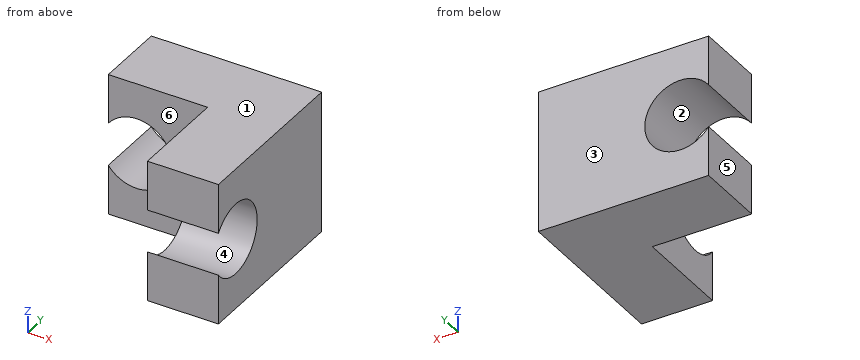
```python
from build123d import *

# Parameters (mm, degrees)
F1_DEPTH       = 12.7
F4_D           = 6.35
F4_DEPTH       = 25.4
F4_TIP         = 1.9077324654
F4_ON_F3_D     = 6.35
F4_ON_F3_DEPTH = 25.4
F4_ON_F3_TIP   = 1.9077324654


with BuildPart() as f1:
    # F0 (on Top) → F1 (new body)
    with BuildSketch(Plane.XY):
        Polygon((-3.6485809102, 10.6884501653), (-3.6485809102, 4.3384501653), (5.2414190898, 4.3384501653), (5.2414190898, -4.5515498347), (11.5914190898, -4.5515498347), (11.5914190898, 10.6884501653), align=None)
    extrude(amount=F1_DEPTH)

    # F4
    with Locations(Plane(origin=(0, 10.6884501653, 0), x_dir=(-1, 0, 0), z_dir=(0, 1, 0))):
        with Locations((1.1085809102, 6.35)):
            Hole(F4_D / 2, depth=F4_DEPTH)
            with Locations((0, 0, -(F4_DEPTH + F4_TIP / 2))):  # 118° drill point
                Cone(0, F4_D / 2, F4_TIP, mode=Mode.SUBTRACT)

    # F4 on F3
    with Locations(Plane.YZ.offset(11.5914190898)):
        with Locations((-2.0115498347, 6.35)):
            Hole(F4_ON_F3_D / 2, depth=F4_ON_F3_DEPTH)
            with Locations((0, 0, -(F4_ON_F3_DEPTH + F4_ON_F3_TIP / 2))):  # 118° drill point
                Cone(0, F4_ON_F3_D / 2, F4_ON_F3_TIP, mode=Mode.SUBTRACT)


solid = f1.part
```
Design review of the part built by this model. Coordinates are the model's own, in mm. Face numbers are marked on the shaded views. A direction names the side the tool comes from. Give positions to 0.01 mm unless a question says otherwise; leave off trailing zeros. Write each loop counter-clockwise with the first axis right and the second up, starting at its lowest first coordinate (ties: lowest second). Pieces come first, ordered by that corner, then holes.
(1) Add section D-D (x = 3). Give the boundary of the cut face in (y, z), and give its area (3 significant figures).
Checked values:
outline: (4.34, 0) - (10.69, 0) - (10.69, 12.7) - (4.34, 12.7) - close
area: 80.6 mm2
(2) Add section B-B (x = 0.75). Give the boundary of the cut face in (y, z).
Checked values:
outline: (4.34, 0) - (10.69, 0) - (10.69, 3.78) - (4.34, 3.78) - close; (4.34, 8.92) - (10.69, 8.92) - (10.69, 12.7) - (4.34, 12.7) - close
(3) Mouldability with a two-part tool opening along Z and no side actions: class the marked faces 1, 2, 3 and 4 as +Z half, -Z half, draft (parallel to the pull), parting line (faces both ways), or undercut.
Checked values:
face 1: +Z half
face 2: undercut
face 3: draft
face 4: undercut
(4) Tool access review of the marked faces 5 and 6: name each direction out of +Z, -Z, +X, -X, +Y, -Y from which nothing blocks a thin tool from reaching the whole face with its end or side.
Checked values:
face 5: +Z, -Z, -X, +Y, -Y
face 6: +Z, -Z, -X, -Y
(5) Add section A-A (z = 2). Give the boundary of the cut face in (x, y).
Checked values:
outline: (-3.65, 4.34) - (5.24, 4.34) - (5.24, -4.55) - (11.59, -4.55) - (11.59, 10.69) - (-3.65, 10.69) - close
(6) Wall thickness on line 1 along X through (y, z) = (-1.25, 9.5); line 2 along Y through (x, z) = (10.25, 6.35); line 3 along Y through (x, z) = (-2.5, 2.75): over which ranges is each line inside the solid? List them lowest first.
Checked values:
line 1: x = 5.24 to 11.59
line 2: y = 1.16 to 10.69
line 3: y = 4.34 to 10.69
(7) Add section C-C (y = 7.25). Give the boundary of the cut face in (x, z) (3 decimals).
Checked values:
outline: (-3.649, 0) - (11.591, 0) - (11.591, 12.7) - (-3.649, 12.7) - (-3.649, 8.255) arc R3.175 cw (long way) to (-3.649, 4.445) - close
(8) Clearance check with flat-ended pins moving along their axes: pin 1 Ø7 at (x, z) = (-0.5, 8) entering from -Y; pin 2 Ø2.5 at (y, z) = (0, 8.5) entering from -X. State where each tip first meets the part, or that it passes through.
Checked values:
pin 1: stops at y = 4.34
pin 2: stops at x = 5.24
